Input: part model. Units: mm. Frame: model coordinates. A direction names the side the tool comes from. Coordinates: 2 decimals unless noted, no trailing zeros. Order: outer loops, then holes, each group sorted by start corner. A loop starts at its lowest first (then second) coordinate and runs counter-clockwise, first axis right, second up. Notation, with made-up numbers: (-7, 74.5) -> (6, 74.5) arc R18 cw to (6, 104.5) -> close; hole circle Ø3 at (-14.5, -2). An arc over 180 degrees is marked (long way). Write each question's results on one line, items separated by ' | '.
```python
from build123d import *

# Parameters (mm, degrees)
SKETCH1_W             = 10
SKETCH1_H             = 40
BOSS_EXTRUDE1_DEPTH   = 3
CAVITY4_START         = 1
CAVITY4_OUTLINE_R     = 2.5
CAVITY4_OUTLINE_R_2   = 0.5
CAVITY4_DEPTH         = 2
CAVITY4_START_2       = 2
CAVITY4_2_OUTLINE_R   = 2.5
CAVITY4_2_OUTLINE_R_2 = 1
CAVITY4_2_DEPTH       = 1
CUT_EXTRUDE4_START    = -23
SKETCH5_R             = 1
CUT_EXTRUDE4_DEPTH    = 23
SKETCH7_W             = 10
SKETCH7_H             = 3
BOSS_EXTRUDE3_DEPTH   = 55
SKETCH8_R             = 1.5
BOSS_EXTRUDE4_DEPTH   = 10
SKETCH9_W             = 10
SKETCH9_H             = 2
BOSS_EXTRUDE5_DEPTH   = 1
FILLET2_R             = 0.5
FILLET3_R             = 0.5


# Read off the part's stored shape, not the designer's step: Cavity4
with BuildPart() as part:
    # Sketch1 → Boss-Extrude1 (new body)
    with BuildSketch(Plane(origin=(0, 0, 0), x_dir=(1, 0, 0), z_dir=(0, 1, 0))):
        with Locations((1.621359223, -14.684466019)):
            Rectangle(SKETCH1_W, SKETCH1_H)
    boss_extrude1 = extrude(amount=BOSS_EXTRUDE1_DEPTH)

    # Cavity4 outline → Cavity4 (cut)
    with BuildSketch(Plane(origin=(0, 0, 0), x_dir=(1, 0, 0), z_dir=(0, 1, 0)).offset(CAVITY4_START)):
        with BuildLine():
            Line((-0.538748891, -15.509698524), (-1.620990225, -27.847249725))
            ThreePointArc((-1.620990225, -27.847249725), (-1.626727223, -27.934549786), (-1.628640777, -28.022017221))
            Line((-1.628640777, -28.022017221), (-1.628640777, -28.045106388))
            ThreePointArc((-1.628640777, -28.045106388), (-1.65149867, -28.346617733), (-1.719549868, -28.641237163))
            ThreePointArc((-1.719549868, -28.641237163), (1.621359223, -33.184466019), (4.962268314, -28.641237163))
            ThreePointArc((4.962268314, -28.641237163), (4.894217117, -28.346617733), (4.871359223, -28.045106388))
            Line((4.871359223, -28.045106388), (4.871359223, -28.022017221))
            ThreePointArc((4.871359223, -28.022017221), (4.86944567, -27.934549786), (4.863708671, -27.847249725))
            Line((4.863708671, -27.847249725), (3.781467338, -15.509698524))
            ThreePointArc((3.781467338, -15.509698524), (3.14012955, -14.209756728), (1.78911789, -13.684466019))
            Line((1.78911789, -13.684466019), (1.453600557, -13.684466019))
            ThreePointArc((1.453600557, -13.684466019), (0.102588897, -14.209756728), (-0.538748891, -15.509698524))
        make_face()
        with Locations((1.621359223, -29.684466019)):
            Circle(CAVITY4_OUTLINE_R, mode=Mode.SUBTRACT)
        with Locations((1.621359223, -25.184466019)):
            Circle(CAVITY4_OUTLINE_R_2, mode=Mode.SUBTRACT)
        with Locations((1.621359223, -23.184466019)):
            Circle(CAVITY4_OUTLINE_R_2, mode=Mode.SUBTRACT)
        with Locations((1.621359223, -21.184466019)):
            Circle(CAVITY4_OUTLINE_R_2, mode=Mode.SUBTRACT)
        with Locations((1.621359223, -19.184466019)):
            Circle(CAVITY4_OUTLINE_R_2, mode=Mode.SUBTRACT)
        with Locations((1.621359223, -17.184466019)):
            Circle(CAVITY4_OUTLINE_R_2, mode=Mode.SUBTRACT)
        with Locations((1.621359223, -15.184466019)):
            Circle(CAVITY4_OUTLINE_R_2, mode=Mode.SUBTRACT)
    extrude(amount=CAVITY4_DEPTH, mode=Mode.SUBTRACT)

    # Cavity4 2 outline → Cavity4 2 (cut)
    with BuildSketch(Plane(origin=(0, 0, 0), x_dir=(1, 0, 0), z_dir=(0, 1, 0)).offset(CAVITY4_START_2)):
        with Locations((1.621359223, -29.684466019)):
            Circle(CAVITY4_2_OUTLINE_R)
        with Locations((1.621359223, -29.684466019)):
            Circle(CAVITY4_2_OUTLINE_R_2, mode=Mode.SUBTRACT)
    extrude(amount=CAVITY4_2_DEPTH, mode=Mode.SUBTRACT)

    # Sketch5 → Cut-Extrude4 (cut)
    with BuildSketch(Plane(origin=(0, 3, 0), x_dir=(1, 0, 0), z_dir=(0, 1, 0)).offset(CUT_EXTRUDE4_START)):
        with Locations(Location((1.621359223, -29.684466019, 0), (0, 0, 270))):
            Circle(SKETCH5_R)
    extrude(amount=CUT_EXTRUDE4_DEPTH, mode=Mode.SUBTRACT)

    # Sketch7 → Boss-Extrude3 (add)
    with BuildSketch(Plane.XZ):
        with Locations((1.621359223, -3.815533981)):
            Rectangle(SKETCH7_W, SKETCH7_H)
    extrude(amount=BOSS_EXTRUDE3_DEPTH)

    # Mirror1: Boss-Extrude1 across plane
    add(boss_extrude1.mirror(Plane(origin=(0, -27.5, 0), x_dir=(0, 0, 1), z_dir=(0, -1, 0))))

    # Sketch8 → Boss-Extrude4 (add)
    with BuildSketch(Plane.XZ.offset(58)):
        with Locations(Location((1.621359223, 29.684466019, 0), (0, 0, 270))):
            Circle(SKETCH8_R)
    extrude(amount=BOSS_EXTRUDE4_DEPTH)

    # Sketch9 → Boss-Extrude5 (add)
    with BuildSketch(Plane.XZ.offset(58)):
        with Locations((1.621359223, -4.315533981)):
            Rectangle(SKETCH9_W, SKETCH9_H)
    boss_extrude5 = extrude(amount=BOSS_EXTRUDE5_DEPTH)

    # Mirror2: Boss-Extrude5 across plane
    add(boss_extrude5.mirror(Plane(origin=(0, -27.5, 0), x_dir=(0, 0, 1), z_dir=(0, -1, 0))))

    # Fillet2
    fillet2_edges = [part.edges().sort_by_distance(p)[0] for p in [
        (6.621359223, 3, 15.684466019),
        (6.621359223, -58, 15.684466019),
    ]]
    fillet(fillet2_edges, radius=FILLET2_R)

    # Fillet3
    fillet3_edges = [part.edges().sort_by_distance(p)[0] for p in [
        (-3.378640777, -58, 15.684466019),
        (-3.378640777, 3, 15.684466019),
    ]]
    fillet(fillet3_edges, radius=FILLET3_R)


solid = part.part
```
(1) Mould query, pull axis Y, two halves, no side actions, for faces 4 (the face through (2, -58, 15)), 5 (the face through (1.6, -58.4, -3.316)), 6 (the face through (2, 3, 11)), 7 (the face through (2, -27, -2.316)). Classes: +Y half, -Y half, draft (parallel to the pull), parting line (faces both ways), or undercut.
Return value:
face 4: -Y half | face 5: draft | face 6: +Y half | face 7: undercut
(2) Cut plane B-B, the plane y = -53. Return loops of the section in (x, z).
Return value:
outline: (-3.38, -5.32) -> (6.62, -5.32) -> (6.62, -2.32) -> (-3.38, -2.32) -> close
(3) Reachability of faces 1 (the face through (2, -28, -5.316)), 2 (the face through (2, -55, 16)), 3 (the face through (1.24, 0.99, 30.61)) from +Z, -Z, +X, -X, +Y, -Y: full face, straight path, thin tool, end or side. Return the list, or none.
Return value:
face 1: -Z, +X, -X, +Y, -Y | face 2: +Z, +X, -X | face 3: +Y
(4) Line query: line 1 along Y through (x, z) = (-2, 7); line 2 along Y through (x, z) = (-0.5, 22.5); line 3 along Z through (x, y) = (3.75, -19). Output: solid intervals per line, ascending. Write a range as from..to.
Return value:
line 1: -58..-55, 0..3 | line 2: -58..-55, 0..1 | line 3: -5.32..-2.32
(5) Cut plane A-A, the plane z = 2.5. Return loops of the section in (x, y).
Return value:
outline: (-3.38, -57.5) arc R0.5 ccw to (-2.88, -58) -> (6.12, -58) arc R0.5 ccw to (6.62, -57.5) -> (6.62, -55) -> (-3.38, -55) -> close; (-3.38, 0) -> (6.62, 0) -> (6.62, 2.5) arc R0.5 ccw to (6.12, 3) -> (-2.88, 3) arc R0.5 ccw to (-3.38, 2.5) -> close
(6) Pin query (flat end, axial travel): P1, Ø10, axis at y = -40.5, z = 5.5, coming from the +X side; P2, Ø3, axis at x = 2.5, y = -22.5, coming from the +Z side; P3, Ø0.8, axis at x = -0.5, y = -58.5, coming from the +Z side; P4, Ø0.5, axis at x = 1.5, z = 21.5, coming from the +Y side. Return the tip coordinate at first contact, or that it passes through.
Return value:
P1: through | P2: z = -2.32 | P3: z = -3.32 | P4: y = 3
